Geometry: see drawing. Coordinates: mm, zero at the bounding-box minimum. A direction names the side the tool comes from. Give positions to 0.01 mm unless a question says otherwise; leave off trailing zeros. Write each loop counter-clockwise with the first axis right and the second up, starting at its lowest first coordinate (ties: lowest second). Pieces come first, ordered by that corner, then holes. Notation, with made-up numbers: (81, 38) - (116, 38) arc R19 ccw to (116, 75) - close; hole circle Ø1 at (5, 47.25). An arc over 180 degrees is marked (long way). Use a Markdown table: item, result. Add a question column.
1. Set-up query: the marked faces 1, 2 and 3. Return all of +Z, -Z, +X, -X, +Y, -Y with unobstructed straight access to the full face (end or side cutting, diameter ignored); none if empty.
2. Section query D-D, the plane z = 12. Return loops of the section in (x, y).
3. Mould query, pull axis Z, two halves, no side actions, for the marked faces 4, 5 and 6. Classes: released by +Z, released by -Z, zero draft, split by the parting line, or undercut.
4. Section query A-A, the plane x = 9.5. Return loops of the section in (y, z).
5. Section query C-C, the plane y = 12.5. Return loops of the section in (x, z), plus the area to 3 significant figures.
6. Pin query (flat end, axial travel): pin 1 (1.5 mm diameter, centred on x = 9, y = 1, fed in from -Z); pin 2 (4 mm diameter, centred on x = 7.5, y = 11, fed in from -Z); pin 3 (4 mm diameter, centred on x = 8.5, z = 11.5, fed in from +Y). Return the tip coordinate at first contact, or that it passes through.
7. Material intervals for probe 1 along X at (y, z) = (14, 12); probe 2 along Z at (x, y) = (10.25, 1.5); probe 3 along Z at (x, y) = (3.25, 8.75), sorted ascending.
8. Section query B-B, the plane z = 5.25. Return loops of the section in (x, y).
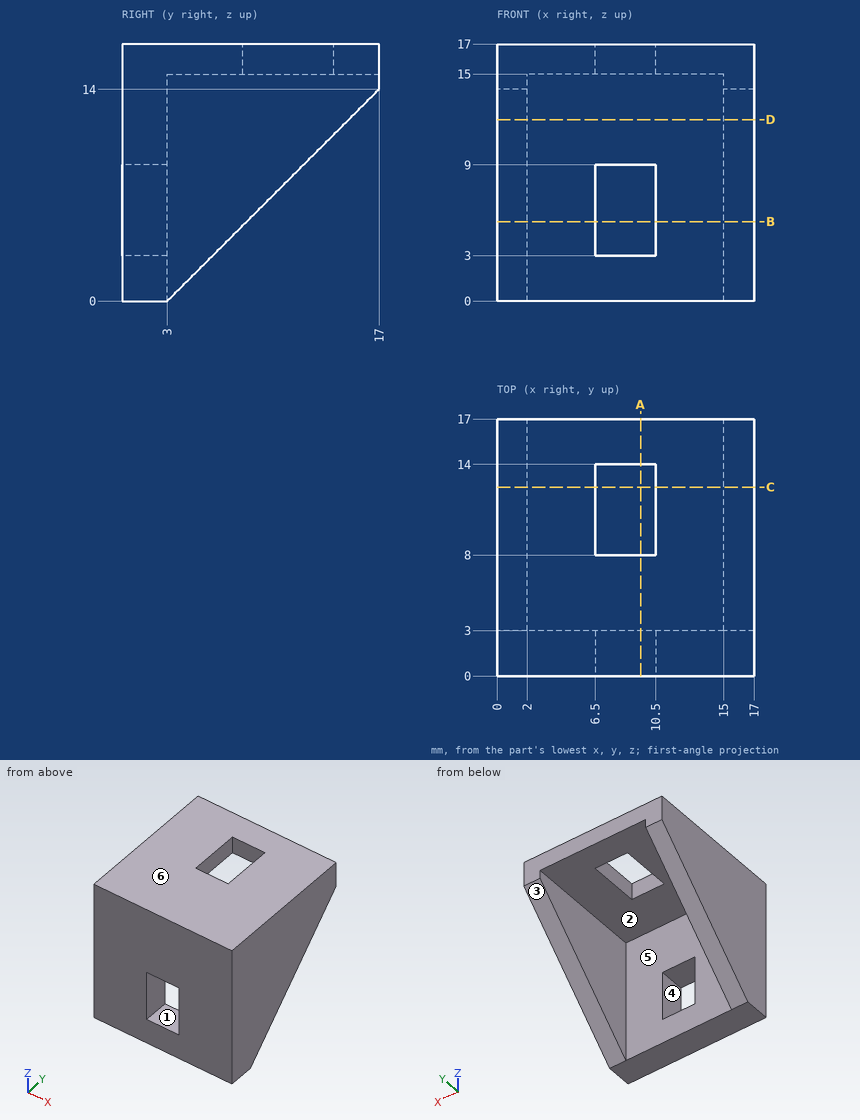
Result sheet:
| question | item | result |
|---|---|---|
| 1 | face 1 | +Y, -Y |
| 1 | face 2 | -Z, +Y |
| 1 | face 3 | -Z, +X, -X, +Y |
| 2 | outline | (0, 0) - (17, 0) - (17, 15) - (15, 15) - (15, 3) - (2, 3) - (2, 15) - (0, 15) - close |
| 3 | face 4 | undercut |
| 3 | face 5 | zero draft |
| 3 | face 6 | released by +Z |
| 4 | outline | (0, 0) - (3, 0) - (3, 3) - (0, 3) - close; (0, 9) - (3, 9) - (3, 15) - (8, 15) - (8, 17) - (0, 17) - close; (14, 15) - (17, 15) - (17, 17) - (14, 17) - close |
| 5 | outline | (0, 9.5) - (2, 9.5) - (2, 15) - (6.5, 15) - (6.5, 17) - (0, 17) - close; (10.5, 15) - (15, 15) - (15, 9.5) - (17, 9.5) - (17, 17) - (10.5, 17) - close |
| 5 | area | 48.0 mm² |
| 6 | pin 1 | stops at z = 0 |
| 6 | pin 2 | stops at z = 15 |
| 6 | pin 3 | stops at y = 3 |
| 7 | probe 1 | x = 0 to 2, 15 to 17 |
| 7 | probe 2 | z = 0 to 3, 9 to 17 |
| 7 | probe 3 | z = 15 to 17 |
| 8 | outline | (0, 0) - (6.5, 0) - (6.5, 3) - (2, 3) - (2, 8.25) - (0, 8.25) - close; (10.5, 0) - (17, 0) - (17, 8.25) - (15, 8.25) - (15, 3) - (10.5, 3) - close |
